Answer from the drawing. Dimensions are ordinates in mm from the lowest x, y and z of the part. A direction names the side the tool comes from. Round coordinates to 2 decimals unless told otherwise and drop trailing zeros. Order: outer loops, then holes, each group sorted by start corner. A loop starts at its lowest first (then second) coordinate and runs counter-clockwise, first axis right, second up. Notation, with made-up numbers: (33.5, 4) -> (80.5, 4) arc R26 cw to (80.5, 40) -> close; hole circle Ø7 at (53.5, 43.25). An arc over 180 degrees is marked (long way). Use a Markdown table: item, result. Add a question column.
Item 1: A cutting plane is placed at D-D, the plane x = 3.75. Determine the outline of the cut face in (y, z).
Item 2: A tool of negligible diameter and unlimited length cuts with its end or side. For the marked faces 4 and 5, from which of +Z, -Z, +X, -X, +Y, -Y can it reach the whole face along a straight path? Write none if from no direction.
Item 3: Find the intervals of material crossed by L1, parallel to Z at x = 9, y = 3; L2, parallel to Y at x = 16.25, z = 9.5; L3, parallel to Z at x = 17, y = 1.95, in increasing order. Write a range as [from, to].
Item 4: For a pull along X with two mould halves and no side action, classify the marked faces 1, 2 and 3 as +X half, -X half, draft (parallel to the pull), parting line (faces both ways), or undercut.
Item 5: A cutting plane is placed at A-A, the plane z = 26.5. Determine the outline of the cut face in (x, y).
Item 6: A cutting plane is placed at C-C, the plane y = 3.7. Determine the outline of the cut face in (x, z), plus the area to 3 significant figures.
Item 7: A cutting plane is placed at B-B, the plane x = 9. Determine the outline of the cut face in (y, z).
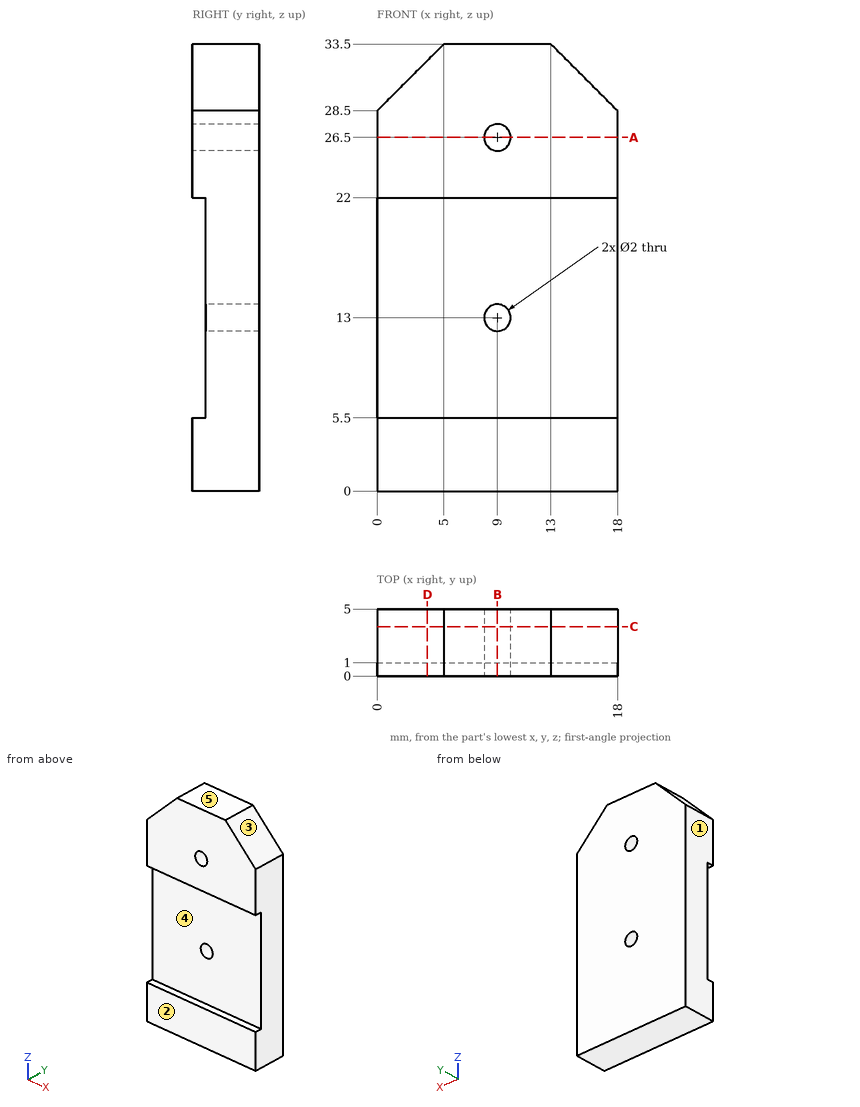
Reported:
| question | item | result |
|---|---|---|
| 1 | outline | (0, 0) -> (5, 0) -> (5, 32.25) -> (0, 32.25) -> (0, 22) -> (1, 22) -> (1, 5.5) -> (0, 5.5) -> close |
| 2 | face 4 | +X, -X, -Y |
| 2 | face 5 | +Z, +X, -X, +Y, -Y |
| 3 | L1 | [0, 12], [14, 25.5], [27.5, 33.5] |
| 3 | L2 | [1, 5] |
| 3 | L3 | [0, 29.5] |
| 4 | face 1 | -X half |
| 4 | face 2 | draft |
| 4 | face 3 | +X half |
| 5 | outline | (0, 0) -> (8, 0) -> (8, 5) -> (0, 5) -> close; (10, 0) -> (18, 0) -> (18, 5) -> (10, 5) -> close |
| 6 | outline | (0, 0) -> (18, 0) -> (18, 28.5) -> (13, 33.5) -> (5, 33.5) -> (0, 28.5) -> close; hole circle Ø2 at (9, 13); hole circle Ø2 at (9, 26.5) |
| 6 | area | 572 mm² |
| 7 | outline | (0, 0) -> (5, 0) -> (5, 12) -> (1, 12) -> (1, 5.5) -> (0, 5.5) -> close; (0, 22) -> (1, 22) -> (1, 14) -> (5, 14) -> (5, 25.5) -> (0, 25.5) -> close; (0, 27.5) -> (5, 27.5) -> (5, 33.5) -> (0, 33.5) -> close |
